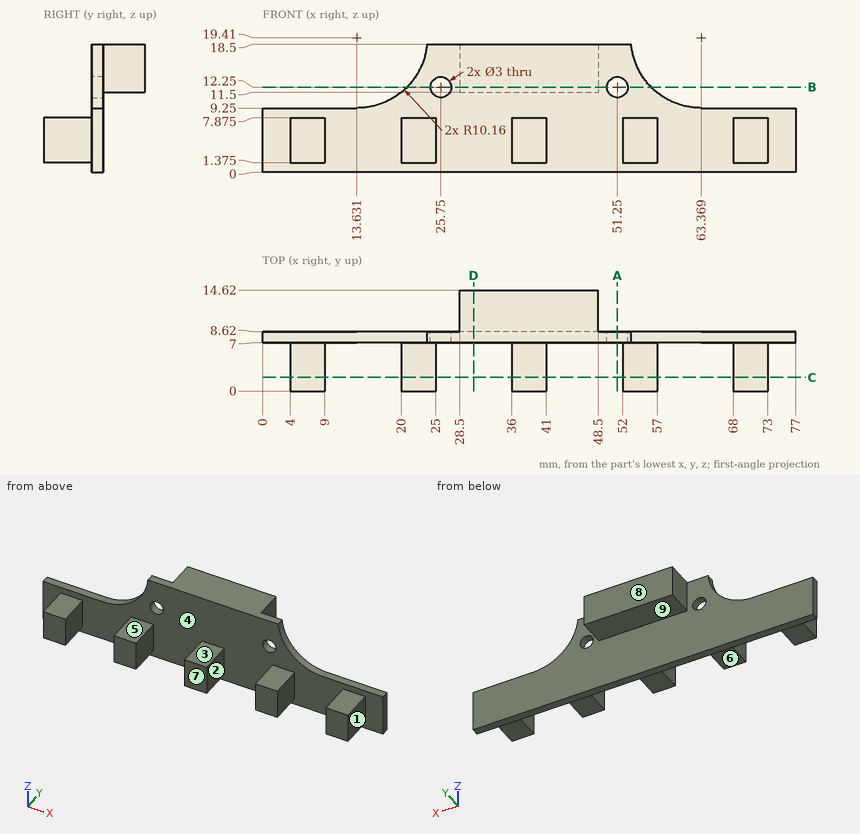
The figure shows three views and two pictorial views of one solid part (mm, origin at its lowest corner). Answer the questions. A direction names the side the tool comes from. Give positions to 0.01 mm unless a question says otherwise; leave off trailing zeros. Loops run counter-clockwise (first coordinate to the right, second up) from the corner with the lowest first, then second, coordinate; pieces in that order, holes last. Notation, with made-up numbers: (-33, 15.25) -> (18, 15.25) arc R15 ccw to (18, 29.25) -> close; hole circle Ø4 at (-32.75, 50.5). An arc over 180 degrees is marked (long way). Put each result on its own line as item: value. Start each with the question number.
Item 1: The mould has two halves that part along X. Classify the marked faces 1, 2, 3 and 4: released by +X, released by -X, zero draft, split by the parting line, or undercut.
Item 2: The part is cut by section C-C (y = 2). Give the vertices of the cut face in (x, z) (3 decimals), then the cut area to 4 significant figures.
Item 3: The part is cut by section B-B (z = 12.25). Give the vertices of the cut face in (x, y).
Item 4: The part is cut by section D-D (x = 30.5). Give the vertices of the cut face in (y, z).
Item 5: Which of the six approach directions +Z, -Z, +X, -X, +Y, -Y give full straight-line access (tool end or side, diameter ignored) to the marked faces 5, 6, 7, 8 and 9?
Item 6: Each of these flat-tipped pins is pushed along its axis until it touches: P1, Ø3.5, axis at x = 25.75, z = 12.25, coming from the +Y side; P2, Ø4, axis at x = 55.5, y = 4, coming from the -Z side (3 decimals); P3, Ø2, axis at y = 3, z = 5.5, coming from the +X side; P4, Ø5, axis at y = 9, z = 4, coming from the +X side. Where does it stop, or does it pass through?
Item 7: Find the intervals of material crossed by L1, parallel to X at y = 3.25, z = 1.5; L2, parallel to X at y = 7.45, z = 12.25; L3, parallel to Z at x = 51.25, y = 8.05, in increasing order. Write a range as [from, to].
Item 8: The part is cut by section A-A (x = 51.25). Give the vertices of the cut face in (y, z), then the cut area to 3 significant figures.
Answers below:
1. face 1: released by +X
1. face 2: undercut
1. face 3: zero draft
1. face 4: undercut
2. outline: (4, 1.375) -> (9, 1.375) -> (9, 7.875) -> (4, 7.875) -> close; (20, 1.375) -> (25, 1.375) -> (25, 7.875) -> (20, 7.875) -> close; (36, 1.375) -> (41, 1.375) -> (41, 7.875) -> (36, 7.875) -> close; (52, 1.375) -> (57, 1.375) -> (57, 7.875) -> (52, 7.875) -> close; (68, 1.375) -> (73, 1.375) -> (73, 7.875) -> (68, 7.875) -> close
2. area: 162.5 mm2
3. outline: (20.84, 7) -> (24.25, 7) -> (24.25, 8.62) -> (20.84, 8.62) -> close; (27.25, 7) -> (49.75, 7) -> (49.75, 8.62) -> (48.5, 8.62) -> (48.5, 14.62) -> (28.5, 14.62) -> (28.5, 8.62) -> (27.25, 8.62) -> close; (52.75, 7) -> (56.16, 7) -> (56.16, 8.62) -> (52.75, 8.62) -> close
4. outline: (7, 0) -> (8.62, 0) -> (8.62, 11.5) -> (14.62, 11.5) -> (14.62, 18.5) -> (7, 18.5) -> close
5. face 5: +Z, +X, -X, -Y
5. face 6: -Z, +X, -X, -Y
5. face 7: +Z, -Z, +X, -X, -Y
5. face 8: +Z, -Z, +X, -X, +Y
5. face 9: -Z, +X, -X, +Y
6. P1: y = 8.62
6. P2: z = 1.375
6. P3: x = 73
6. P4: x = 77
7. L1: [4, 9], [20, 25], [36, 41], [52, 57], [68, 73]
7. L2: [20.84, 24.25], [27.25, 49.75], [52.75, 56.16]
7. L3: [0, 10.75], [13.75, 18.5]
8. outline: (7, 0) -> (8.62, 0) -> (8.62, 10.75) -> (7, 10.75) -> close; (7, 13.75) -> (8.62, 13.75) -> (8.62, 18.5) -> (7, 18.5) -> close
8. area: 25.1 mm2
